Build history of the part. All positions in model axes, mm. Give positions to 0.01 mm unless a question says otherwise; leave off trailing zeros. Loops run counter-clockwise (first coordinate to the right, second up) from the corner with the lowest first, then second, coordinate; pieces in that order, holes last. Notation, with made-up numbers: M -11,67.5 L 21,67.5 A15 ccw 21,96.5 Z; hole C -0.75,4 d4. An arc over 180 degrees is marked long. Answer as a JSON object with one key per item and string values. Group by question number.
1. Drop flat-ended pins along their axis: pin 1 Ø12 at (x, y) = (8.5, -8.5) entering from +Z; pin 2 Ø1 at (x, z) = (49.5, 0.5) entering from -Y; pin 3 Ø0.6 at (x, z) = (-20, 0.5) entering from -Y; pin 4 Ø2.5 at (x, y) = (44.75, 44.18) entering from +Z. Give the stop position or say it passes through.
2. Drill centre lines: line 1 along Y through (x, z) = (-40.5, 1.75); line 2 along X through (y, z) = (-8.5, 1.35); line 3 along X through (y, z) = (-23, 0.6). Where is each one in solid material? Low to high. Write a range as [from, to].
3. Slice it at A-A (y = 24). List the corners of the cut face in (x, z), then the cut area to 3 significant figures.
4. Slice it at D-D (y = -31). List the corners of the cut face in (x, z).
5. Slice it at B-B (x = -10.5). Give the number of separate pieces and of enclosed holes in the cut face, then the cut area to 3 significant figures.
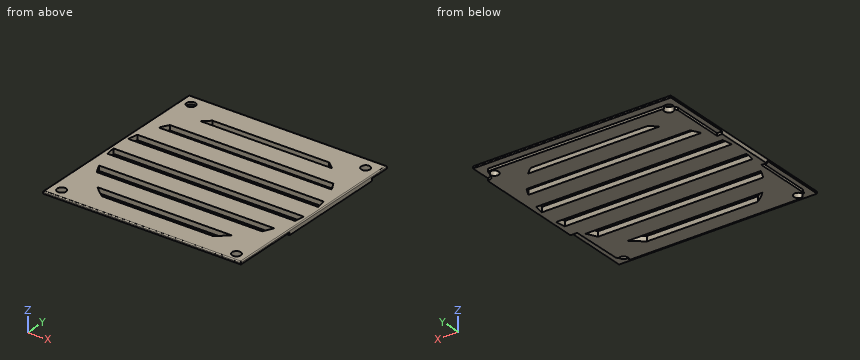
from build123d import *

# Parameters (mm, degrees)
F0_W      = 101.6
F0_H      = 101.6
F0_R      = 50.2793
F1_DEPTH  = 2.54
F3_DEPTH  = 2.541
F5_DEPTH  = 1.27
F6_R      = 0.508
F7_R      = 2.286
F8_DEPTH  = 2.541
F9_R      = 2.286
F10_DEPTH = 2.541


with BuildPart() as f1:
    # F0 (on Top) → F1 (new body)
    with BuildSketch(Plane.XY):
        Rectangle(F0_W, F0_H)
        Circle(F0_R, mode=Mode.SUBTRACT)
        Circle(F0_R)
    extrude(amount=F1_DEPTH)

    # F2 (on face) → F3 (cut, through all)
    with BuildSketch(Plane.XY.offset(2.54)):
        with BuildLine():
            Line((-33.768142, 35.632432), (33.768142, 35.632432))
            ThreePointArc((33.768142, 35.632432), (31.879279, 37.331879), (29.905016, 38.931319))
            Line((29.905016, 38.931319), (-29.905016, 38.931319))
            ThreePointArc((-29.905016, 38.931319), (-31.879279, 37.331879), (-33.768142, 35.632432))
        make_face()
        with BuildLine():
            Line((-44.373298, 20.999238), (44.373298, 20.999238))
            ThreePointArc((44.373298, 20.999238), (43.227357, 23.266999), (41.965615, 25.472432))
            Line((41.965615, 25.472432), (-41.965615, 25.472432))
            ThreePointArc((-41.965615, 25.472432), (-43.227357, 23.266999), (-44.373298, 20.999238))
        make_face()
        with BuildLine():
            Line((-48.752321, 5.759238), (48.752321, 5.759238))
            ThreePointArc((48.752321, 5.759238), (48.382744, 8.310698), (47.87973, 10.839238))
            Line((47.87973, 10.839238), (-47.87973, 10.839238))
            ThreePointArc((-47.87973, 10.839238), (-48.382744, 8.310698), (-48.752321, 5.759238))
        make_face()
        with BuildLine():
            Line((48.167134, -9.480762), (48.893669, -4.400762))
            Line((48.893669, -4.400762), (-48.893669, -4.400762))
            ThreePointArc((-48.893669, -4.400762), (-48.596826, -6.950262), (-48.167134, -9.480762))
            Line((-48.167134, -9.480762), (48.167134, -9.480762))
        make_face()
        with BuildLine():
            Line((42.412752, -24.720762), (44.991089, -19.640762))
            Line((44.991089, -19.640762), (-44.991089, -19.640762))
            ThreePointArc((-44.991089, -19.640762), (-43.775672, -22.218194), (-42.412752, -24.720762))
            Line((-42.412752, -24.720762), (42.412752, -24.720762))
        make_face()
        with BuildLine():
            Line((28.514823, -39.960762), (34.544031, -34.880762))
            Line((34.544031, -34.880762), (-34.544031, -34.880762))
            ThreePointArc((-34.544031, -34.880762), (-31.631572, -37.541993), (-28.514823, -39.960762))
            Line((-28.514823, -39.960762), (28.514823, -39.960762))
        make_face()
    extrude(amount=-F3_DEPTH, mode=Mode.SUBTRACT)

    # F4 (on face) → F5 (cut)
    with BuildSketch(Plane(origin=(0, 0, 0), x_dir=(1, 0, 0), z_dir=(0, 0, -1))):
        Polygon((-48.20291, 44.609038), (-45.037047, 48.350511), (43.894938, 48.350511), (47.060798, 43.457819), (47.348599, 16.979685), (50.8, 16.979685), (50.8, 50.8), (-50.8, 50.8), (-50.8, 15.97322), (-48.20291, 15.540657), align=None)
        Polygon((-48.167134, -15.109803), (-50.8, -15.109803), (-50.8, -50.8), (50.8, -50.8), (50.8, -40.436711), (48.167134, -41.300129), (45.905016, -47.056243), (-44.991089, -46.768438), (-48.167134, -42.451348), align=None)
    extrude(amount=-F5_DEPTH, mode=Mode.SUBTRACT)

    # F6
    f6_edges = [f1.edges().sort_by_distance(p)[0] for p in [
        (0, 50.8, 2.54),
        (-50.8, 0, 2.54),
        (0, -50.8, 2.54),
        (50.8, 0, 2.54),
    ]]
    fillet(f6_edges, radius=F6_R)

    # F7 (on face) → F8 (cut, through all)
    with BuildSketch(Plane.XY.offset(2.54)):
        with Locations((-45.329407, 44.753794)):
            Circle(F7_R)
        with Locations((44.753794, 44.178184)):
            Circle(F7_R)
        with Locations((45.204923, -46.339341)):
            Circle(F7_R)
    extrude(amount=-F8_DEPTH, mode=Mode.SUBTRACT)

    # F9 (on face) → F10 (cut, through all)
    with BuildSketch(Plane.XY.offset(2.54)):
        with Locations((-45.041602, -45.617212)):
            Circle(F9_R)
    extrude(amount=-F10_DEPTH, mode=Mode.SUBTRACT)


solid = f1.part
Established:
{
 "1": {"pin 1": "stops at z = 2.54", "pin 2": "stops at y = -16.98", "pin 3": "stops at y = -48.35", "pin 4": "passes through"},
 "2": {"line 1": "y = [-50.8, -24.72], [-19.64, -9.48], [-4.4, 5.76], [10.84, 21], [25.47, 50.8]", "line 2": "x = [-50.8, -48.35], [48.31, 50.8]", "line 3": "x = [-48.2, -43.37], [43.29, 47.28]"},
 "3": {"outline": "M -50.8,1.27 L -48.17,1.27 L -48.17,0 L -42.82,0 L -42.82,2.54 L -50.29,2.54 A0.51 ccw -50.8,2.03 Z; M 42.82,0 L 50.8,0 L 50.8,2.03 A0.51 ccw 50.29,2.54 L 42.82,2.54 Z", "area": "37.1 mm^2"},
 "4": {"outline": "M -50.8,1.27 L -48.2,1.27 L -48.2,0 L 47.2,0 L 47.2,1.27 L 50.8,1.27 L 50.8,2.03 A0.51 ccw 50.29,2.54 L -50.29,2.54 A0.51 ccw -50.8,2.03 Z"},
 "5": {"separate pieces": "7", "enclosed holes": "0", "area": "179 mm^2"}
}
